Input: part model. Units: mm. Frame: model coordinates. Give positions to 0.01 mm unless a question says otherwise; leave off trailing zeros. Answer in a Markdown table with one row per item. Add a question column.
Solid Edge part; units mm, degrees
sketch "Sketch1" plane through (0, 0, 0) normal (0, -1, 0) x (1, 0, 0)
  line L0 (0, 1.05) -> (0, -4.5126)
  arc A0 (-0.076, 1.9182) -> (0, 1.05) centre (-5, 1.05) cw
  line L1 (-4.0896, 24.6806) -> (-0.076, 1.9182)
  arc A1 (-4.0896, 24.6806) -> (-3.864, 27.2589) centre (0.8345, 25.5488) cw
  line L2 (-3.864, 27.2589) -> (-2.7312, 30.3715)
sketch "Sketch2" plane through (0, 0, -4.5126) normal (0, 0, -1) x (-1, 0, 0)
  circle A0 centre (0, 0) radius 1.25
sweep "SweptProtrusion_2" add profiles "Sketch2" path "Sketch1"
sketch "Sketch3" plane through (0, 0, 0) normal (0, -1, 0) x (1, 0, 0)
  line L0 (0, 1.05) -> (0, -4.5126)
  arc A0 (-0.076, 1.9182) -> (0, 1.05) centre (-5, 1.05) cw
  line L1 (-4.0896, 24.6806) -> (-0.076, 1.9182)
  arc A1 (-4.0896, 24.6806) -> (-3.864, 27.2589) centre (0.8345, 25.5488) cw
  line L2 (-3.864, 27.2589) -> (-2.7312, 30.3715)
sketch "Sketch4" plane through (0, 0, -4.5126) normal (0, 0, -1) x (-1, 0, 0)
  circle A0 centre (0, 0) radius 0.75
sweep "SweptCutout_1" cut profiles "Sketch4" path "Sketch3"
sketch "Sketch5" plane through (0, 0, 0) normal (0, -1, 0) x (1, 0, 0)
  line L0 (-3.9058, 30.799) -> (-2.6894, 26.8314)
extrude "ExtrudedCutout_1" cut sketch "Sketch5" along normal mid plane 7.6718 material side at (-3.2498, 0, 28.8299)
properties material "Galvanized steel"
Q1. Line query: probe 1 along Y at (x, z) = (0, -2.2); probe 2 along X at (y, z) = (0.3, 8); probe 3 along Y at (x, z) = (-3.25, 27.5). Output: solid intervals per line, ascending.
Q2. Pull-direction query (Y, two-part tool) for faces 1 (the cylindrical face through (0.75, 0.03, -1.77)), 2 (the cylindrical face through (0.27, -1.22, -1.77)), 3 (the flat face through (-1, 0, -4.513)); classes: +Y half, -Y half, draft (parallel to the pull), parting line (faces both ways), or undercut.
Q3. Contact query for flat-ended pins moving along their axis: P1, Ø1, axis at y = -0.5, z = 8.5, coming from the +X side; P2, Ø1, axis at y = -0.5, z = 20.5, coming from the +X side. Output: stop coordinate, or through.
Computed:
| question | item | result |
|---|---|---|
| 1 | probe 1 | y = -1.25 to -0.75, 0.75 to 1.25 |
| 1 | probe 2 | x = -2.38 to -1.85, -0.45 to 0.08 |
| 1 | probe 3 | y = -1.15 to -0.56, 0.56 to 1.15 |
| 2 | face 1 | undercut |
| 2 | face 2 | parting line |
| 2 | face 3 | draft |
| 3 | P1 | stops at x = 0.09 |
| 3 | P2 | stops at x = -2.03 |
